Read the model definition and answer for the solid it produces. Units are mm, in the model's axes. A direction names the side the tool comes from. Round coordinates to 2 decimals unless told otherwise and drop trailing zeros. Loops run counter-clockwise (first coordinate to the right, second up) from the corner with the lowest first, then second, coordinate; pieces in that order, holes last. Notation, with made-up numbers: (51, 37) -> (56, 37) arc R28 ccw to (56, 58) -> close; hole circle Ø4 at (14, 59.5). An arc over 180 degrees is marked (long way). Put each result on its own line as item: value.
from build123d import *

# Parameters (mm, degrees)
F0_R     = 15
F0_R_2   = 4
F1_DEPTH = 12
F0_R_3   = 17
F2_DEPTH = 2
F3_R     = 17
F3_R_2   = 15
F4_DEPTH = 2


with BuildPart() as f1:
    # F0 (on Top) → F1 (new body)
    with BuildSketch(Plane.XY):
        Circle(F0_R)
        Circle(F0_R_2, mode=Mode.SUBTRACT)
    extrude(amount=F1_DEPTH)

    # F0 (on Top) → F2 (join)
    with BuildSketch(Plane.XY):
        Circle(F0_R_3)
        Circle(F0_R, mode=Mode.SUBTRACT)
    extrude(amount=F2_DEPTH)

    # F3 (on face) → F4 (join)
    with BuildSketch(Plane.XY.offset(12)):
        Circle(F3_R)
        Circle(F3_R_2, mode=Mode.SUBTRACT)
    extrude(amount=-F4_DEPTH)


solid = f1.part
Item 1: The part is cut by section A-A (x = 0). Determine the outline of the cut face in (y, z), then the cut area to 3 significant figures.
Derived:
outline: (-17, 0) -> (-4, 0) -> (-4, 12) -> (-17, 12) -> (-17, 10) -> (-15, 10) -> (-15, 2) -> (-17, 2) -> close; (4, 0) -> (17, 0) -> (17, 2) -> (15, 2) -> (15, 10) -> (17, 10) -> (17, 12) -> (4, 12) -> close
area: 280 mm^2
Item 2: Flat-ended cylindrical pins translate along their axes: pin 1 Ø3 at (y, z) = (-12, 9) entering from +X; pin 2 Ø3 at (y, z) = (-7, 1.5) entering from -X; pin 3 Ø6 at (x, z) = (-8.5, 2) entering from +Y. Find the tip coordinate at first contact, or state that the pin passes through.
Derived:
pin 1: stops at x = 13.06
pin 2: stops at x = -16.09
pin 3: stops at y = 16.09
Item 3: Which of the six approach directions +Z, -Z, +X, -X, +Y, -Y give full straight-line access (tool end or side, diameter ignored) to faces 1 (the flat face through (4, -4, 0)), 2 (the cylindrical face through (-14.985, 0.66, 5.944))?
Derived:
face 1: -Z, +X, -X, +Y, -Y
face 2: none
Item 4: The part is cut by section C-C (x = -5). Determine the outline of the cut face in (y, z), then the cut area to 3 significant figures.
Derived:
outline: (-16.25, 0) -> (16.25, 0) -> (16.25, 2) -> (14.14, 2) -> (14.14, 10) -> (16.25, 10) -> (16.25, 12) -> (-16.25, 12) -> (-16.25, 10) -> (-14.14, 10) -> (-14.14, 2) -> (-16.25, 2) -> close
area: 356 mm^2
Item 5: For a pull along Z with two mould halves and no side action, classify faces 3 (the flat face through (4, -4, 12)), 4 (the flat face through (6, -14, 2)), 5 (the cylindrical face through (9.139, 14.334, 0.986)) as pulls with the +Z half, pulls with the -Z half, needs draft (parallel to the pull), parting line crosses it, or undercut.
Derived:
face 3: pulls with the +Z half
face 4: undercut
face 5: needs draft
Item 6: The part is cut by section D-D (y = 14.5). Determine the outline of the cut face in (x, z), then the cut area to 3 significant figures.
Derived:
outline: (-8.87, 0) -> (8.87, 0) -> (8.87, 2) -> (3.84, 2) -> (3.84, 10) -> (8.87, 10) -> (8.87, 12) -> (-8.87, 12) -> (-8.87, 10) -> (-3.84, 10) -> (-3.84, 2) -> (-8.87, 2) -> close
area: 132 mm^2
Item 7: Find the intervals of material crossed by line 1 along Y through (x, z) = (0, 2.5); line 2 along Z through (x, y) = (-1.5, -15); line 3 along X through (y, z) = (-3, 1.75), in increasing order.
Derived:
line 1: y = -15 to -4, 4 to 15
line 2: z = 0 to 2, 10 to 12
line 3: x = -16.73 to -2.65, 2.65 to 16.73
